Here's the drawing with two shaded views (mm, measured from the low corner). I have some questions. Coordinates: 2 decimals unless noted, no trailing zeros. Write each loop counter-clockwise with the first axis right and the second up, starting at its lowest first coordinate (ties: lowest second). Pieces come first, ordered by that corner, then holes. Notation, with made-up numbers: M 75.25,78.25 L 109.25,78.25 A21 cw 109.25,108.25 Z; hole C -16,-17 d3. An arc over 180 degrees is marked long. Answer as CSV lines item,"result". Start each with the question number.
Item 1: Suppose I cut it at C-C, the plane z = 9.5. State how many separate pieces and enclosed holes the cut face has, and give its area (3 significant figures).
Item 2: We'd pull the mould along X, two halves only. Please class the marked faces 1, 2 and 3: +X half, -X half, draft (parallel to the pull), parting line (faces both ways), or undercut.
Item 3: Suppose I cut it at D-D, the plane y = 24. Write out the boundary of the cut face in (x, z) (1 decimal).
Item 4: If I drill on line 1 along X through (y, z) = (21, 7.5) (1 decimal); line 2 along X through (y, z) = (19, 2.25); line 3 along Y through (x, z) = (33, 10), over which ranges is the centre line in solid material (lowest first)? Write a range as [from, to].
Item 5: Suppose I cut it at B-B, the plane x = 11. Write out the boundary of the cut face in (y, z).
Item 6: Suppose I cut it at A-A, the plane y = 32.5. Write out the boundary of the cut face in (x, z), and give its area (3 significant figures).
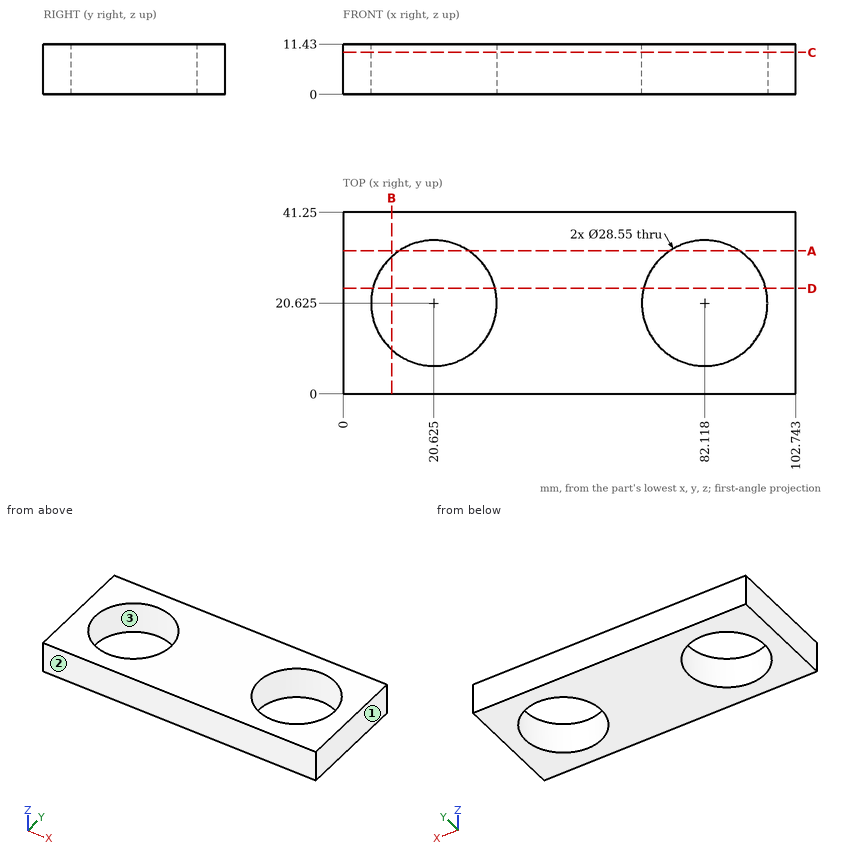
Ans:
1,separate pieces,"1"
1,enclosed holes,"2"
1,area,"2,960 mm^2"
2,face 1,"+X half"
2,face 2,"draft"
2,face 3,"undercut"
3,outline,"M 0,0 L 6.8,0 L 6.8,11.4 L 0,11.4 Z; M 34.5,0 L 68.2,0 L 68.2,11.4 L 34.5,11.4 Z; M 96,0 L 102.7,0 L 102.7,11.4 L 96,11.4 Z"
4,line 1,"x = [0, 6.4], [34.9, 67.8], [96.4, 102.7]"
4,line 2,"x = [0, 6.44], [34.81, 67.94], [96.3, 102.74]"
4,line 3,"y = [0, 13.51], [27.74, 41.25]"
5,outline,"M 0,0 L 10.08,0 L 10.08,11.43 L 0,11.43 Z; M 31.17,0 L 41.25,0 L 41.25,11.43 L 31.17,11.43 Z"
6,outline,"M 0,0 L 12.7,0 L 12.7,11.43 L 0,11.43 Z; M 28.55,0 L 74.2,0 L 74.2,11.43 L 28.55,11.43 Z; M 90.04,0 L 102.74,0 L 102.74,11.43 L 90.04,11.43 Z"
6,area,"812 mm^2"
